The figure shows three views and two pictorial views of one solid part (mm, origin at its lowest corner). Answer the questions. Coordinates: 2 decimals unless noted, no trailing zeros. Write each loop counter-clockwise with the first axis right and the second up, starting at its lowest first coordinate (ties: lowest second). Pieces come first, ordered by that corner, then holes.
Item 1: Section B-B (z = 5.25) is taken. Give the vertices of the cut face in (x, y), then the cut area to 3 significant figures.
Item 2: Straight lines are drawn through the part: probe 1 along X at (y, z) = (1.5, 7.5); probe 2 along Z at (x, y) = (40, 1.05); probe 3 along X at (y, z) = (1.1, 5). For each, find the intervals that lie inside material, in ascending order.
Item 3: Section A-A (x = 10) is taken. Give the vertices of the cut face in (y, z).
Item 4: Section D-D (z = 10) is taken. Give the vertices of the cut face in (x, y).
Item 5: Section C-C (y = 0.8) is taken. Give the vertices of the cut face in (x, z).
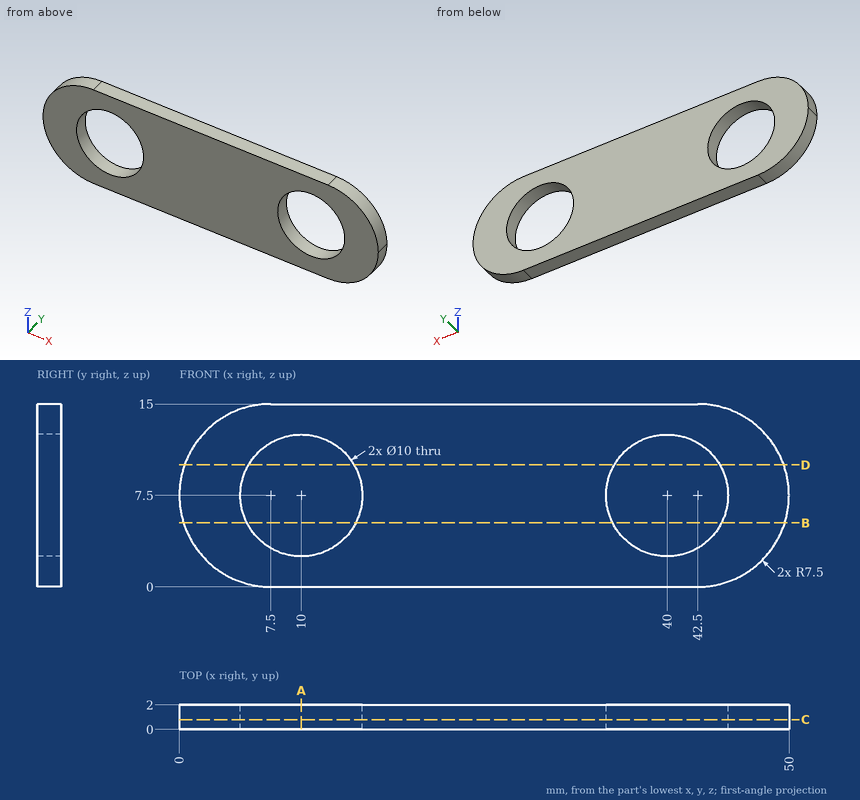
Established:
1. outline: (0.35, 0) - (5.53, 0) - (5.53, 2) - (0.35, 2) - close; (14.47, 0) - (35.53, 0) - (35.53, 2) - (14.47, 2) - close; (44.47, 0) - (49.65, 0) - (49.65, 2) - (44.47, 2) - close
1. area: 62.9 mm2
2. probe 1: x = 0 to 5, 15 to 35, 45 to 50
2. probe 2: z = 0 to 2.5, 12.5 to 15
2. probe 3: x = 0.43 to 5.67, 14.33 to 35.67, 44.33 to 49.57
3. outline: (0, 0) - (2, 0) - (2, 2.5) - (0, 2.5) - close; (0, 12.5) - (2, 12.5) - (2, 15) - (0, 15) - close
4. outline: (0.43, 0) - (5.67, 0) - (5.67, 2) - (0.43, 2) - close; (14.33, 0) - (35.67, 0) - (35.67, 2) - (14.33, 2) - close; (44.33, 0) - (49.57, 0) - (49.57, 2) - (44.33, 2) - close
5. outline: (7.5, 0) - (42.5, 0) arc R7.5 ccw to (42.5, 15) - (7.5, 15) arc R7.5 ccw to start; hole circle Ø10 at (10, 7.5); hole circle Ø10 at (40, 7.5)
